Check sheet for the modelled part. Datum: model origin and axes. Units: mm. Face numbers are marked on the shaded views. A direction names the side the tool comes from. Give positions to 0.01 mm unless a question says otherwise; leave off trailing zeros. Write each loop counter-clockwise with the first axis right and the second up, starting at its lowest first coordinate (ties: lowest second). Pieces come first, ordered by that corner, then holes. Notation, with made-up numbers: M 72.25,-18 L 129.25,-18 A31 cw 129.25,13 Z; hole C 79,16.5 d10. An arc over 180 degrees is marked long. One line per item, written item: value. Start each with the question number.
from build123d import *

# Parameters (mm, degrees)
F1_DEPTH = 63.5
F0_W     = 25.4
F0_H     = 19.0499988828
F0_H_2   = 4.7498011172
F0_H_3   = 4.7752
F2_DEPTH = 25.4
F3_DEPTH = 7.9375
F4_R     = 6.35


with BuildPart() as f1:
    # F0 (on Front) → F1 (new body, symmetric)
    with BuildSketch(Plane.XZ):
        Polygon((-41.275, 9.525), (-41.275, -9.525), (41.275, -9.525), (41.275, 9.525), (22.2250011172, 9.525), align=None)
    extrude(amount=F1_DEPTH, both=True)

    # F0 (on Front) → F2 (join, symmetric)
    with BuildSketch(Plane.XZ):
        with BuildLine():
            Line((22.2250011172, 9.525), (41.275, 9.525))
            Line((41.275, 9.525), (41.275, 27.0002))
            ThreePointArc((41.275, 27.0002), (45.9246798487, 38.2255201513), (57.15, 42.8752))
            Line((57.15, 42.8752), (60.325, 42.8752))
            Line((60.325, 42.8752), (60.325, 61.9251988828))
            Line((60.325, 61.9251988828), (57.15, 61.9251988828))
            ThreePointArc((57.15, 61.9251988828), (32.454296457, 51.695903543), (22.2250011172, 27.0002))
            Line((22.2250011172, 27.0002), (22.2250011172, 9.525))
        make_face()
        with Locations((73.025, 52.4001994414)):
            Rectangle(F0_W, F0_H)
        with Locations((73.025, 64.3000994414)):
            Rectangle(F0_W, F0_H_2)
        with Locations((73.025, 40.4876)):
            Rectangle(F0_W, F0_H_3)
    extrude(amount=F2_DEPTH, both=True)

    # F0 (on Front) → F3 (join, symmetric)
    with BuildSketch(Plane.XZ):
        with BuildLine():
            add(Edge.make_bspline(
                [(-41.275, 9.525), (-31.7300852137, 44.8146195103), (19.3697411857, 62.6715747871), (57.15, 61.9251988828)],
                knots=[0, 0, 0, 0, 111.5045356385, 111.5045356385, 111.5045356385, 111.5045356385], degree=3))
            Line((-41.275, 9.525), (22.2250011172, 9.525))
            Line((22.2250011172, 9.525), (22.2250011172, 27.0002))
            ThreePointArc((22.2250011172, 27.0002), (32.454296457, 51.695903543), (57.15, 61.9251988828))
        make_face()
    extrude(amount=F3_DEPTH, both=True)

    # F4
    f4_edges = [f1.edges().sort_by_distance(p)[0] for p in [
        (-41.275, -63.5, 0),
        (41.275, -63.5, 0),
        (41.275, 63.5, 0),
        (-41.275, 63.5, 0),
    ]]
    fillet(f4_edges, radius=F4_R)


solid = f1.part
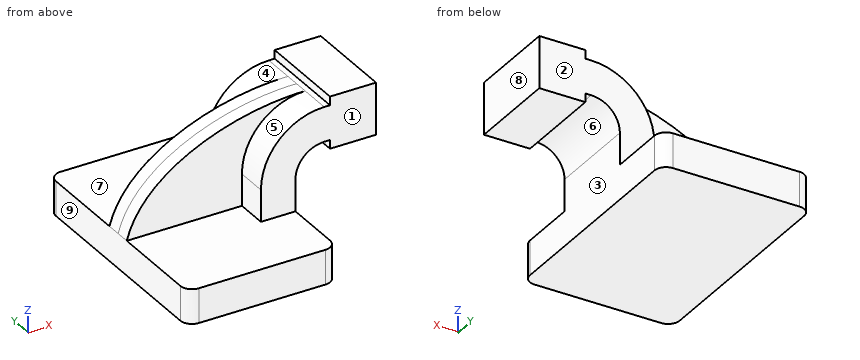
1) Material ranges on L1, parallel to Z at x = 76, y = -12 (3 decimals); L2, parallel to Z at x = -24, y = -22.5 (3 decimals); L3, parallel to Y at x = 20, z = 45.5, recorded low to high. Write a range as from..to.
2) Cross-section at C-C (y = 45). Record the boundary of the cut face in (x, z) (3 decimals), plus the area to 3 significant figures.
3) Tool access check on the marked faces 1, 2, 3, 4 and 5. Record the directions out of +Z, -Z, +X, -X, +Y, -Y that give a thin tool (end or side, any length) a straight path to the whole face; none if there is none.
4) Cross-section at B-B (z = -5). Record the boundary of the cut face in (x, y) (3 decimals).
5) Gauge pin test, flat ends, axial feed: pin 1 (18.5 mm diameter, centred on y = 15, z = 0.5, fed in from +X) (3 decimals); pin 2 (17 mm diameter, centred on x = 43, z = 33.5, fed in from -Y); pin 3 (14 mm diameter, centred on y = 15.5, z = 20, fed in from -X) (3 decimals). Record the tip position at first contact, or that the pin passes through.
6) Draft check along X on the marked faces 6, 7, 8 and 9. Enter one of: released by +X, released by -X, zero draft, split by the parting line, or undercut.
7) Cross-section at A-A (y = -11). Record the boundary of the cut face in (x, z) (3 decimals).
Data:
1. L1: z = 38.1..66.675
1. L2: z = -9.525..9.525
1. L3: y = -7.94..7.94
2. outline: M -41.275,-9.525 L 41.275,-9.525 L 41.275,9.525 L -41.275,9.525 Z
2. area: 1,570 mm2
3. face 1: +Z, +X, -X, -Y
3. face 2: +Z, +X, -X, +Y
3. face 3: -Z, +X, +Y, -Y
3. face 4: +Z, -X, +Y
3. face 5: +Z, -X, -Y
4. outline: M -41.275,-57.15 A6.35 ccw -34.925,-63.5 L 34.925,-63.5 A6.35 ccw 41.275,-57.15 L 41.275,57.15 A6.35 ccw 34.925,63.5 L -34.925,63.5 A6.35 ccw -41.275,57.15 Z
5. pin 1: stops at x = 41.275
5. pin 2: stops at y = -25.4
5. pin 3: stops at x = 22.225
6. face 6: undercut
6. face 7: zero draft
6. face 8: released by +X
6. face 9: released by -X
7. outline: M -41.275,-9.525 L 41.275,-9.525 L 41.275,27 A15.875 cw 57.15,42.875 L 60.325,42.875 L 60.325,38.1 L 85.725,38.1 L 85.725,66.675 L 60.325,66.675 L 60.325,61.925 L 57.15,61.925 A34.925 ccw 22.225,27 L 22.225,9.525 L -41.275,9.525 Z
